from build123d import *

# Parameters (mm, degrees)
SKETCH1_R           = 12.5
BOSS_EXTRUDE1_DEPTH = 15
SCALE1_SCALE        = 1.9329
SCALE2_SCALE        = 1.5
SKETCH3_R           = 40.633377722
BOSS_EXTRUDE2_DEPTH = 12.1499924
SKETCH4_R           = 36.241875
BOSS_EXTRUDE3_DEPTH = 50
SKETCH5_R           = 36.241875
BOSS_EXTRUDE4_DEPTH = 71


with BuildPart() as part:
    # Sketch1 → Boss-Extrude1 (new body)
    with BuildSketch(Plane(origin=(0, 0, 0), x_dir=(0, 0, -1), z_dir=(1, 0, 0))):
        Circle(SKETCH1_R)
    extrude(amount=BOSS_EXTRUDE1_DEPTH)


with BuildPart() as part_1:
    # Scale1: scaled about (7.5, 0, 0)
    add(part.part.scale(SCALE1_SCALE).moved(Location((-6.99675, 0, 0))))


with BuildPart() as part_2:
    # Scale2: scaled about (7.5, 0, 0)
    add(part_1.part.scale(SCALE2_SCALE).moved(Location((-3.75, 0, 0))))

    # Sketch3 → Boss-Extrude2 (add)
    with BuildSketch(Plane(origin=(29.245125, 0, 0), x_dir=(0, 0, -1), z_dir=(1, 0, 0))):
        Circle(SKETCH3_R)
    extrude(amount=BOSS_EXTRUDE2_DEPTH)

    # Sketch4 → Boss-Extrude3 (add)
    with BuildSketch(Plane(origin=(41.3951174, 0, 0), x_dir=(0, 0, -1), z_dir=(1, 0, 0))):
        Circle(SKETCH4_R)
    extrude(amount=BOSS_EXTRUDE3_DEPTH)

    # Sketch5 → Boss-Extrude4 (add)
    with BuildSketch(Plane(origin=(91.3951174, 0, 0), x_dir=(0, 0, -1), z_dir=(1, 0, 0))):
        Circle(SKETCH5_R)
    extrude(amount=BOSS_EXTRUDE4_DEPTH)


solid = part_2.part
Read the model definition and answer for the solid it produces. Units are mm, in the model's axes. A direction names the side the tool comes from. Round coordinates to 2 decimals unless told otherwise and drop trailing zeros. Write each loop counter-clockwise with the first axis right and the second up, starting at its lowest first coordinate (ties: lowest second). Pieces come first, ordered by that corner, then holes.
Q1. Flat-ended cylindrical pins translate along their axes: P1, Ø5, axis at x = 38, y = 19.5, coming from the +Z side; P2, Ø3, axis at x = 11.5, y = 15, coming from the +Z side; P3, Ø2, axis at x = 11.5, z = -14, coming from the -Y side. Find the tip coordinate at first contact, or state that the pin passes through.
Values:
P1: stops at z = 36.91
P2: stops at z = 33.63
P3: stops at y = -33.83
Q2. Straight lines are drawn through the part: line 1 (Z direction, x = 61, y = 0.5); line 2 (X direction, y = 35.5, z = -18.5); line 3 (Y direction, x = 103, z = 31). For each, find the intervals that lie inside material, in ascending order.
Values:
line 1: z = -36.24 to 36.24
line 2: x = 29.25 to 41.4
line 3: y = -18.77 to 18.77
Q3. A tool of negligible diameter and unlimited length cuts with its end or side. For faces 1 (the face through (101.05, -22.05, 28.76)), 2 (the face through (35.235, -15.563, -37.535)), 3 (the face through (7.2, -22.05, 28.76)), from which of +Z, -Z, +X, -X, +Y, -Y can it reach the whole face along a straight path? Write none if from no direction.
Values:
face 1: +X
face 2: +X, -X
face 3: -X
Q4. Find section A-A on y = 0. Determine the outline of the cut face in (x, z), and give its area (3 significant figures).
Values:
outline: (-14.25, -36.24) - (29.25, -36.24) - (29.25, -40.63) - (41.4, -40.63) - (41.4, -36.24) - (162.4, -36.24) - (162.4, 36.24) - (41.4, 36.24) - (41.4, 40.63) - (29.25, 40.63) - (29.25, 36.24) - (-14.25, 36.24) - close
area: 12,900 mm2
Q5. Find section C-C on x = 83. Determine the outline of the cut face in (y, z).
Values:
outline: circle Ø72.48 at (0, 0)
